```python
from build123d import *

# Parameters (mm, degrees)
CUT_EXTRUDE_1_DEPTH = 1.5
FILLET_1_R          = 0.3
CHAMFER_1_SIZE      = 1


with BuildPart() as part:
    # Эскиз1 → Повернуть1 (revolve)
    with BuildSketch(Plane.XY):
        with BuildLine():
            Line((0, 0), (0, 3.625))
            ThreePointArc((0, 3.625), (0.908821487, 4.451033224), (2.1, 4.75))
            Line((2.1, 4.75), (2.6, 4.75))
            Line((2.6, 4.75), (2.6, 2.5))
            Line((2.6, 2.5), (22.6, 2.5))
            Line((22.6, 2.5), (22.6, 0))
            Line((22.6, 0), (0, 0))
        make_face()
    revolve(axis=Axis((22.6, 0, 0), (-1, 0, 0)))

    # Эскиз2 → Вырез-Вытянуть1 (cut)
    with BuildSketch(Plane.ZY):
        Polygon((0.866025404, 1.5), (-0.866025404, 1.5), (-1.732050808, 0), (-0.866025404, -1.5), (0.866025404, -1.5), (1.732050808, 0), align=None)
    extrude(amount=-CUT_EXTRUDE_1_DEPTH, mode=Mode.SUBTRACT)

    # Скругление1
    fillet_1_edges = [part.edges().sort_by_distance(p)[0] for p in [
        (2.6, -2.5, 0),
        (2.6, -4.75, 0),
    ]]
    fillet(fillet_1_edges, radius=FILLET_1_R)

    # Фаска1
    chamfer_1_edges = [part.edges().sort_by_distance(p)[0] for p in [
        (22.6, -2.5, 0),
    ]]
    chamfer(chamfer_1_edges, length=CHAMFER_1_SIZE)


solid = part.part
```
Read the model definition and answer for the solid it produces. Units are mm, in the model's axes. A direction names the side the tool comes from. Coordinates: 2 decimals unless noted, no trailing zeros. Order: outer loops, then holes, each group sorted by start corner. A loop starts at its lowest first (then second) coordinate and runs counter-clockwise, first axis right, second up. Notation, with made-up numbers: (66, 80) - (116, 80) arc R18 ccw to (116, 93) - close; hole circle Ø3 at (62, 36). An arc over 180 degrees is marked (long way). Answer as a JSON object with one key per item and string values. Group by question number.
Item 1: Section A-A (x = 10.25) is taken. Give the vertices of the cut face in (y, z), plus the area to 3 significant figures.
Item 2: A tool of negligible diameter and unlimited length cuts with its end or side. For faces 4 (the face through (22.6, 0, 0)), 5 (the face through (1.5, 0, 0)), 6 (the face through (2.6, 0, 3)), from which of +Z, -Z, +X, -X, +Y, -Y can it reach the whole face along a straight path? Write none if from no direction.
Item 3: Flat-ended cylindrical pins translate along their axes: P1, Ø1.5, axis at x = 18, z = -1.5, coming from the +Y side; P2, Ø1.5, axis at y = -0.5, z = -0.5, coming from the -X side; P3, Ø1.5, axis at x = 10, z = -2.5, coming from the -Y side. Find the tip coordinate at first contact, or state that the pin passes through.
Item 4: The mould has two halves that part along Z. Classify faces 1 (the face through (12.38, -0.54, 2.44)), 2 (the face through (0, -2, 0)), 3 (the face through (0.74, 0.76, -1.293)): +Z half, -Z half, draft (parallel to the pull), parting line (faces both ways), or undercut.
Item 5: Consider probe 1 along X at (y, z) = (1, 0.5); probe 2 along X at (y, z) = (-1, -3); probe 3 along Y at (x, z) = (8.25, 2). Determine where each line is inside the solid, lowest interval first. Write a range as from..to.
Results are:
{
 "1": {"outline": "circle Ø5 at (0, 0)", "area": "19.6 mm^2"},
 "2": {"face 4": "+Z, -Z, +X, +Y, -Y", "face 5": "-X", "face 6": "+X"},
 "3": {"P1": "stops at y = 2.38", "P2": "stops at x = 1.5", "P3": "stops at y = -1.79"},
 "4": {"face 1": "parting line", "face 2": "draft", "face 3": "undercut"},
 "5": {"probe 1": "x = 1.5..22.6", "probe 2": "x = 0..2.6", "probe 3": "y = -1.5..1.5"}
}
